Verification items for the finished model (mm, model axes). Face numbers are marked on the shaded views. A direction names the side the tool comes from. Coordinates: 2 decimals unless noted, no trailing zeros. Loops run counter-clockwise (first coordinate to the right, second up) from the corner with the lowest first, then second, coordinate; pieces in that order, holes last. Notation, with made-up numbers: (21, -31) - (37, -31) arc R18 cw to (37, -8) - close; hole circle Ø10 at (64.5, 55.5). An arc over 180 degrees is marked (long way). One line per item, written item: value. Start each with the question number.
(1) Set-up check for the marked faces 1 and 2: record each of +Z, -Z, +X, -X, +Y, -Y from which the full face is reachable in a straight line by a thin tool's end or side.
(2) Draft check along Z on the marked faces 3, 4, 5 and 6. Enter one of: +Z half, -Z half, draft (parallel to the pull), parting line (faces both ways), or undercut.
(3) Section check C-C (z = 47.5). Record the boundary of the cut face in (x, y).
(4) Section check A-A (y = -280.5). Record the boundary of the cut face in (x, z).
(5) Gauge pin test, flat ends, axial feed: P1, Ø10, axis at y = -106, z = 136.5, coming from the +X side; P2, Ø6, axis at y = -119.5, z = 19.5, coming from the +X side. Record the tip position at first contact, or that the pin passes through.
(6) Section check B-B (x = 516). Record the boundary of the cut face in (y, z), plus the area to 3 significant figures.
(7) Thickness scan on probe 1 along Z at (x, y) = (53.5, -96); probe 2 along X at (y, z) = (-211, 108.5); probe 3 along Y at (x, z) = (231, 132). Record the ranges inside material, lowest first. Write a range as [from, to].
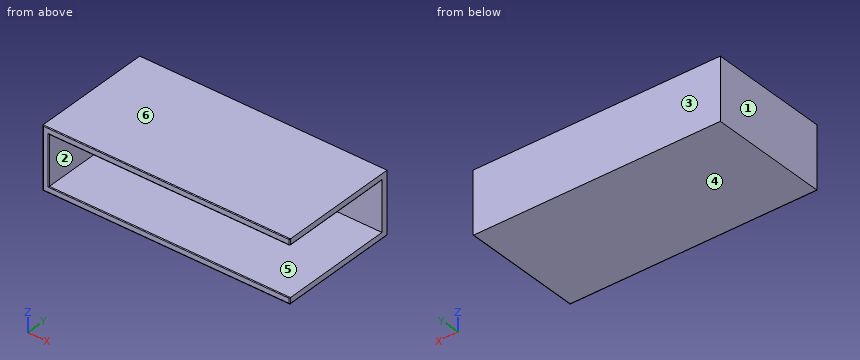
```python
from build123d import *

# Parameters (mm, degrees)
F0_W     = 51.6054928303
F0_H     = 42.5849854946
F1_DEPTH = 350
F2_DEPTH = 718
F3_DEPTH = 180
F4_T     = -18
F5_R     = 2


# Not quite as in the source:
# - two fillets or chamfers of one size are made in one step


with BuildPart() as f1:
    # F0 (on Front) → F1 (new body)
    with BuildSketch(Plane.XZ):
        with Locations((25.8027464151, 21.2924927473)):
            Rectangle(F0_W, F0_H)
    extrude(amount=F1_DEPTH)

    # F2 (add): a face of the model
    f2_faces = [f1.faces().sort_by_distance(p)[0] for p in [
        (0, -175, 21.2924927473),
    ]]
    extrude(f2_faces, amount=-F2_DEPTH)

    # F3 (add): a face of the model
    f3_faces = [f1.faces().sort_by_distance(p)[0] for p in [
        (359, -175, 0),
    ]]
    extrude(f3_faces, amount=-F3_DEPTH)

    # F4
    f4_openings = [f1.faces().sort_by_distance(p)[0] for p in [
        (359, -350, 90),
        (718, -175, 90),
    ]]
    offset(amount=F4_T, openings=f4_openings)

    # F5
    f5_edges = [f1.edges().sort_by_distance(p)[0] for p in [
        (359, -350, 180),
        (0, -350, 90),
        (359, -350, 0),
        (718, -175, 0),
        (718, -350, 9),
        (368, -350, 18),
        (18, -350, 90),
        (368, -350, 162),
        (718, -350, 171),
        (718, -184, 162),
    ]]
    fillet(f5_edges, radius=F5_R)


solid = f1.part
```
Responses:
1. face 1: +Z, -Z, -X, +Y, -Y
1. face 2: +X, -Y
2. face 3: draft
2. face 4: -Z half
2. face 5: undercut
2. face 6: +Z half
3. outline: (0, -348) arc R2 ccw to (2, -350) - (16, -350) arc R2 ccw to (18, -348) - (18, -18) - (718, -18) - (718, 0) - (0, 0) - close
4. outline: (0, 0) - (716, 0) arc R2 ccw to (718, 2) - (718, 18) - (18, 18) - (18, 162) - (716, 162) arc R2 ccw to (718, 164) - (718, 180) - (0, 180) - close
5. P1: stops at x = 18
5. P2: stops at x = 718
6. outline: (-350, 2) arc R2 ccw to (-348, 0) - (0, 0) - (0, 180) - (-348, 180) arc R2 ccw to (-350, 178) - (-350, 164) arc R2 ccw to (-348, 162) - (-18, 162) - (-18, 18) - (-348, 18) arc R2 ccw to (-350, 16) - close
6. area: 15,200 mm²
7. probe 1: z = [0, 18], [162, 180]
7. probe 2: x = [0, 18]
7. probe 3: y = [-18, 0]
